Geometry: final body of the model. Coordinates: model frame, mm. A direction names the side the tool comes from. Coordinates: 2 decimals unless noted, no trailing zeros. Order: outer loops, then holes, each group sorted by start corner. A loop starts at its lowest first (then second) coordinate and runs counter-clockwise, first axis right, second up. Notation, with made-up numbers: (0, 51) -> (6, 51) arc R24 cw to (6, 79) -> close; hole circle Ø3 at (15, 32.5). An arc over 180 degrees is marked (long way). Answer in a Markdown table with one row per item. Add a question column.
1) Section query D-D on x = 7. Return the cut outline in (y, z), then the cut area to 3 significant figures.
2) Set-up query: faces 5 (the face through (14, 0, -25)), 6 (the face through (34.5, 18.66, -12.62)). Return all of +Z, -Z, +X, -X, +Y, -Y with unobstructed straight access to the full face (end or side cutting, diameter ignored); none if empty.
3) Pull-direction query (X, two-part tool) for faces 1 (the face through (0, 6, -25)), 2 (the face through (50, 6, -25)), 3 (the face through (27.688, 12.675, -16.463)), 4 (the face through (25, 6, -50)); classes: +X half, -X half, draft (parallel to the pull), parting line (faces both ways), or undercut.
4) Ray query, line 1 (X direction, y = 6.25, z = -25); line 2 (X direction, y = 13.5, z = -25) (3 decimals); line 3 (Z direction, x = 25.5, y = 2.5). Return the intervals inside material, ascending. Write a range as from..to.
5) Contact query for flat-ended pins moving along their axis: P1, Ø4, axis at x = 44.5, z = -17, coming from the +Y side; P2, Ø3, axis at x = 32, y = 14.5, coming from the +Z side; P3, Ø1.5, axis at x = 30, y = 19, coming from the -Z side. Output: stop coordinate, or through.
6) Section query A-A on x = 25. Return the cut outline in (y, z) (3 decimals), then the cut area to 3 significant figures.
7) Section query C-C on y = 7.75. Return the cut outline in (x, z).
8) Section query B-B on z = -25. Return the cut outline in (x, y) (3 decimals), then the cut area to 3 significant figures.
```python
from build123d import *

# Parameters (mm, degrees)
SKETCH1_W           = 50
SKETCH1_H           = 50
BOSS_EXTRUDE1_DEPTH = 12.5
SKETCH2_R           = 15.605
SKETCH2_R_2         = 8.95
BOSS_EXTRUDE2_DEPTH = 12.5
SKETCH3_R           = 8.95
CUT_EXTRUDE1_DEPTH  = 76


with BuildPart() as part:
    # Sketch1 → Boss-Extrude1 (new body)
    with BuildSketch(Plane(origin=(0, 0, 0), x_dir=(1, 0, 0), z_dir=(0, 1, 0))):
        with Locations((25, 25)):
            Rectangle(SKETCH1_W, SKETCH1_H)
    extrude(amount=BOSS_EXTRUDE1_DEPTH)

    # Sketch2 → Boss-Extrude2 (add)
    with BuildSketch(Plane(origin=(0, 12.5, 0), x_dir=(1, 0, 0), z_dir=(0, 1, 0))):
        with Locations(Location((25, 25, 0), (0, 0, 90))):
            Circle(SKETCH2_R)
        with Locations(Location((25, 25, 0), (0, 0, 270))):
            Circle(SKETCH2_R_2, mode=Mode.SUBTRACT)
    extrude(amount=BOSS_EXTRUDE2_DEPTH)

    # Sketch3 → Cut-Extrude1 (cut, through all)
    with BuildSketch(Plane(origin=(0, 25, 0), x_dir=(1, 0, 0), z_dir=(0, 1, 0))):
        with Locations(Location((25, 25, 0), (0, 0, 270))):
            Circle(SKETCH3_R)
    extrude(amount=-CUT_EXTRUDE1_DEPTH, mode=Mode.SUBTRACT)


solid = part.part
```
Result:
| question | item | result |
|---|---|---|
| 1 | outline | (0, -50) -> (12.5, -50) -> (12.5, 0) -> (0, 0) -> close |
| 1 | area | 625 mm2 |
| 2 | face 5 | +Z, -Z, +X, -X, -Y |
| 2 | face 6 | +Y |
| 3 | face 1 | -X half |
| 3 | face 2 | +X half |
| 3 | face 3 | undercut |
| 3 | face 4 | draft |
| 4 | line 1 | 0..16.05, 33.95..50 |
| 4 | line 2 | 9.395..16.05, 33.95..40.605 |
| 4 | line 3 | -50..-33.94, -16.06..0 |
| 5 | P1 | y = 12.5 |
| 5 | P2 | z = -10.4 |
| 5 | P3 | z = -40.02 |
| 6 | outline | (0, -50) -> (12.5, -50) -> (12.5, -40.605) -> (25, -40.605) -> (25, -33.95) -> (0, -33.95) -> close; (0, -16.05) -> (25, -16.05) -> (25, -9.395) -> (12.5, -9.395) -> (12.5, 0) -> (0, 0) -> close |
| 6 | area | 568 mm2 |
| 7 | outline | (0, -50) -> (50, -50) -> (50, 0) -> (0, 0) -> close; hole circle Ø17.9 at (25, -25) |
| 8 | outline | (0, 0) -> (16.05, 0) -> (16.05, 25) -> (9.395, 25) -> (9.395, 12.5) -> (0, 12.5) -> close; (33.95, 0) -> (50, 0) -> (50, 12.5) -> (40.605, 12.5) -> (40.605, 25) -> (33.95, 25) -> close |
| 8 | area | 568 mm2 |
